Autodesk Inventor part; units mm, degrees
ref_plane "to_magnet_XY" through (0, 1.6, 0) normal (0, -1, 0) x (1, 0, 0)
ref_plane "to_magnet_YZ" through (0, 1.6, 0) normal (1, 0, 0) x (0, 0, 1)
ref_plane "to_magnet_ZX" through (0, 1.6, 0) normal (0, 0, 1) x (0, -1, 0)
sketch "Sketch_1" plane through (0, 0, 0) normal (0, 0, 1) x (1, 0, 0)
  line L0 (-15, 0) -> (15, 0)
  line L1 (15, 0) -> (15, 1.6)
  line L2 (15, 1.6) -> (-15, 1.6)
  line L3 (-15, 1.6) -> (-15, 0)
extrude "Extrusion1" add sketch "Sketch_1" along normal mid plane 16
sketch "Sketch_2" plane through (0, 0, 0) normal (0, 0, 1) x (1, 0, 0)
  line L0 (8, 0) -> (8, 1.6)
  line L1 (8, 1.6) -> (11.1, 1.6)
  line L2 (11.1, 1.6) -> (11.1, 1.5)
  line L3 (11.1, 1.5) -> (9.6, 0)
  line L4 (9.6, 0) -> (8, 0)
  line L5 (8, 0) -> (8, 1.6)
revolve "Revolution1" cut sketch "Sketch_2" angle 360 about axis through (8, 0, 0) along (0, -1, 0)
sketch "Sketch_3" plane through (0, 0, 0) normal (0, 0, 1) x (1, 0, 0)
  line L0 (-8, 0) -> (-8, 1.6)
  line L1 (-8, 1.6) -> (-4.9, 1.6)
  line L2 (-4.9, 1.6) -> (-4.9, 1.5)
  line L3 (-4.9, 1.5) -> (-6.4, 0)
  line L4 (-6.4, 0) -> (-8, 0)
  line L5 (-8, 0) -> (-8, 1.6)
revolve "Revolution2" cut sketch "Sketch_3" angle 360 about axis through (-8, 0, 0) along (0, -1, 0)
ref_plane "to_magnet_XY" through (0, 1.6, 0) normal (0, -1, 0) x (1, 0, 0)
ref_plane "to_magnet_YZ" through (0, 1.6, 0) normal (1, 0, 0) x (0, 0, 1)
ref_plane "to_magnet_ZX" through (0, 1.6, 0) normal (0, 0, 1) x (0, -1, 0)
ref_plane "to_bolt1_XY" through (-8, 0.1, 0) normal (0, 1, 0) x (1, 0, 0)
ref_plane "to_bolt1_YZ" through (-8, 0.1, 0) normal (1, 0, 0) x (0, 0, -1)
ref_plane "to_bolt1_ZX" through (-8, 0.1, 0) normal (0, 0, -1) x (0, 1, 0)
ref_plane "to_bolt2_XY" through (8, 0.1, 0) normal (0, 1, 0) x (1, 0, 0)
ref_plane "to_bolt2_YZ" through (8, 0.1, 0) normal (1, 0, 0) x (0, 0, -1)
ref_plane "to_bolt2_ZX" through (8, 0.1, 0) normal (0, 0, -1) x (0, 1, 0)
properties part number "MGCE1plate5-5"
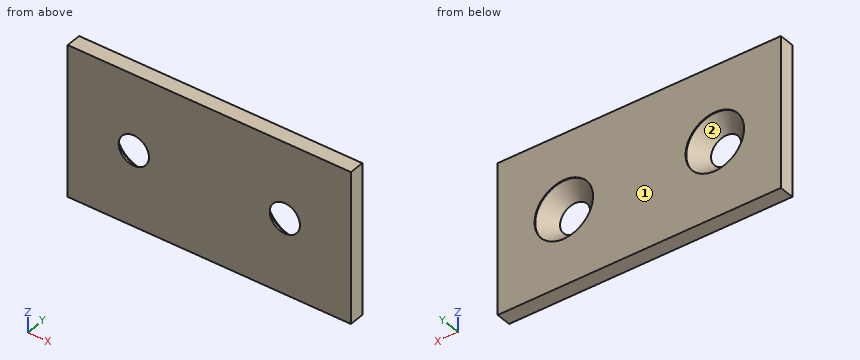
Here's how the part is built. I have some questions about the finished solid (model axes, mm). Face numbers are marked on the shaded views. Coordinates: 2 decimals unless noted, no trailing zeros. Order: outer loops, then holes, each group sorted by start corner. A loop starts at its lowest first (then second) coordinate and runs counter-clockwise, first axis right, second up. Notation, with made-up numbers: (-25, 61.5) - (28, 61.5) arc R4 ccw to (28, 66.5) - close; hole circle Ø7 at (69.25, 25.25). An arc over 180 degrees is marked (long way). Use CSV: the item, a comma, the result in double quotes. Start each with the question number.
1. I'm going to push a flat-ended pin straight in: pin 1 (6 mm diameter, centred on x = -9, z = 2.5, fed in from +Y). Where does the tip first touch, or does it pass through?
2. If we mould it in two halves opening along Z, with no side actions, what happens to the marked faces 1 and 2? For each: +Z half, -Z half, draft (parallel to the pull), parting line (faces both ways), or undercut.
3. Suppose I cut it at A-A on x = 8. List the corners of the cut face in (y, z) for me, then the cut area to 3 significant figures.
4. Suppose I cut it at B-B on z = 0. List the corners of the cut face in (x, y) for me, then the cut area to 3 significant figures.
5. Please list where these lines run through material, in increasing order: line 1 (Z direction, x = 9.25, y = 0.45); line 2 (X direction, y = 0.4, z = 1.25); line 3 (Z direction, x = 6.75, y = 0.2). Write a range as from..to.
6. Suppose I cut it at C-C on y = 0.6. List the corners of the cut face in (x, z) for me.
Output:
1,pin 1,"stops at y = 1.6"
2,face 1,"draft"
2,face 2,"undercut"
3,outline,"(0, -8) - (1.6, -8) - (1.6, -3.1) - (1.5, -3.1) - (0, -1.6) - close; (0, 1.6) - (1.5, 3.1) - (1.6, 3.1) - (1.6, 8) - (0, 8) - close"
3,area,"17.9 mm2"
4,outline,"(-15, 0) - (-9.6, 0) - (-11.1, 1.5) - (-11.1, 1.6) - (-15, 1.6) - close; (-6.4, 0) - (6.4, 0) - (4.9, 1.5) - (4.9, 1.6) - (-4.9, 1.6) - (-4.9, 1.5) - close; (9.6, 0) - (15, 0) - (15, 1.6) - (11.1, 1.6) - (11.1, 1.5) - close"
4,area,"32.7 mm2"
5,line 1,"z = -8..-1.62, 1.62..8"
5,line 2,"x = -15..-9.56, -6.44..6.44, 9.56..15"
5,line 3,"z = -8..-1.3, 1.3..8"
6,outline,"(-15, -8) - (15, -8) - (15, 8) - (-15, 8) - close; hole circle Ø4.4 at (-8, 0); hole circle Ø4.4 at (8, 0)"
